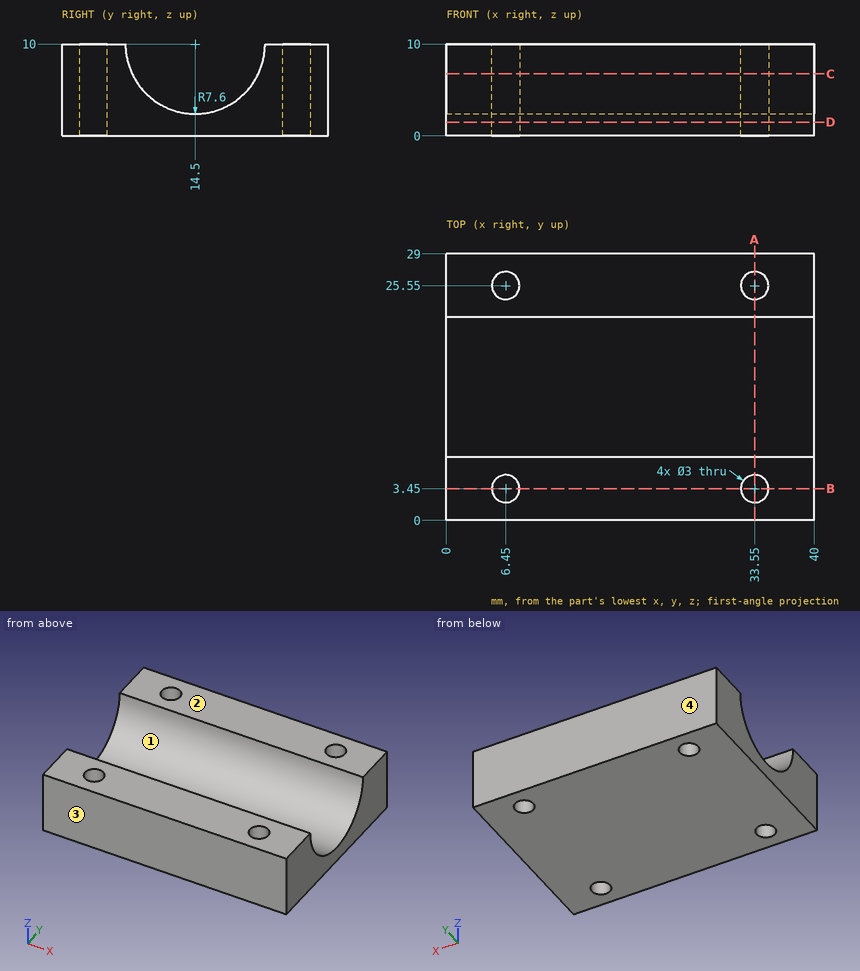
The figure shows three views and two pictorial views of one solid part (mm, origin at its lowest corner). Answer the questions. Round coordinates to 2 decimals unless told otherwise and drop trailing zeros. Loops run counter-clockwise (first coordinate to the right, second up) from the corner with the lowest first, then second, coordinate; pieces in that order, holes last. Notation, with made-up numbers: (45, -17) -> (49, -17) arc R12 ccw to (49, 5) -> close; hole circle Ø3 at (60.25, -13.75). An arc over 180 degrees is marked (long way). Use one line per item in the form item = value.
(1) Find section D-D on z = 1.5. Give the vertices of the cut face in (x, y).
Answer list:
outline = (0, 0) -> (40, 0) -> (40, 29) -> (0, 29) -> close; hole circle Ø3 at (6.45, 3.45); hole circle Ø3 at (6.45, 25.55); hole circle Ø3 at (33.55, 3.45); hole circle Ø3 at (33.55, 25.55)
(2) Straight lines are drawn through the part: line 1 (X direction, y = 3.5, z = 5.5); line 2 (Y direction, x = 6, z = 6); line 3 (X direction, y = 26.5, z = 3.5). For each, find the intervals that lie inside material, in ascending order.
Answer list:
line_1 = 0 to 4.95, 7.95 to 32.05, 35.05 to 40
line_2 = 0 to 2.02, 4.88 to 8.04, 20.96 to 24.12, 26.98 to 29
line_3 = 0 to 5.29, 7.61 to 32.39, 34.71 to 40
(3) Find section B-B on y = 3.45. Give the vertices of the cut face in (x, z).
Answer list:
outline = (0, 0) -> (4.95, 0) -> (4.95, 10) -> (0, 10) -> close; (7.95, 0) -> (32.05, 0) -> (32.05, 10) -> (7.95, 10) -> close; (35.05, 0) -> (40, 0) -> (40, 10) -> (35.05, 10) -> close
(4) Find section A-A on x = 33.55. Give the vertices of the cut face in (y, z).
Answer list:
outline = (0, 0) -> (1.95, 0) -> (1.95, 10) -> (0, 10) -> close; (4.95, 0) -> (24.05, 0) -> (24.05, 10) -> (22.1, 10) arc R7.6 cw to (6.9, 10) -> (4.95, 10) -> close; (27.05, 0) -> (29, 0) -> (29, 10) -> (27.05, 10) -> close
(5) For a pull along Y with two mould halves and no side action, classify the marked faces 1, 2, 3 and 4 as released by +Y, released by -Y, zero draft, split by the parting line, or undercut.
Answer list:
face_1 = undercut
face_2 = zero draft
face_3 = released by -Y
face_4 = released by +Y
(6) Find section C-C on z = 6.75. Give the vertices of the cut face in (x, y), then the cut area to 3 significant figures.
Answer list:
outline = (0, 0) -> (40, 0) -> (40, 7.63) -> (0, 7.63) -> close; (0, 21.37) -> (40, 21.37) -> (40, 29) -> (0, 29) -> close; hole circle Ø3 at (6.45, 3.45); hole circle Ø3 at (6.45, 25.55); hole circle Ø3 at (33.55, 3.45); hole circle Ø3 at (33.55, 25.55)
area = 582 mm2
(7) Flat-ended cylindrical pins translate along their axes: P1, Ø2.5, axis at x = 6.45, y = 25.55, coming from the -Z side; P2, Ø1.5, axis at x = 24, y = 19, coming from the +Z side. Find the tip coordinate at first contact, or state that the pin passes through.
Answer list:
P1 = through
P2 = 4.5
